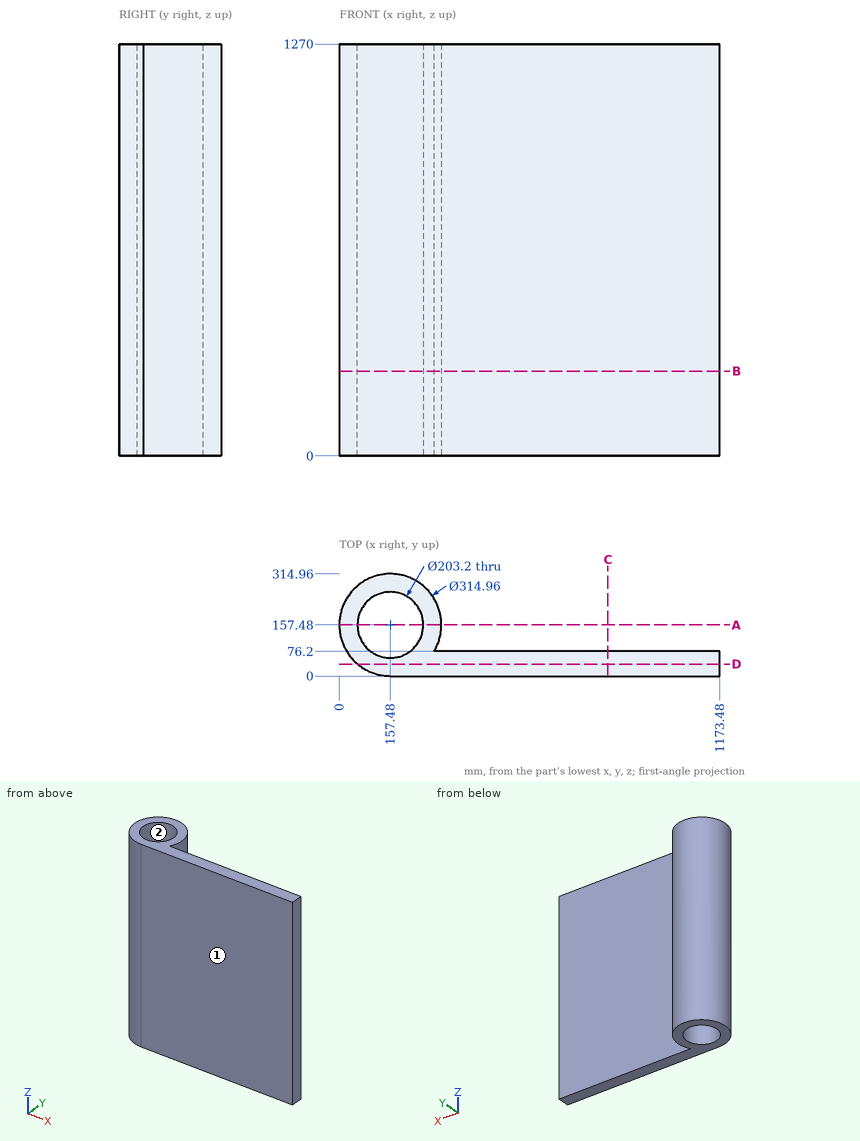
Here's the drawing with two shaded views (mm, measured from the low corner). I have some questions. Coordinates: 2 decimals unless noted, no trailing zeros. Order: outer loops, then holes, each group sorted by start corner. A loop starts at its lowest first (then second) coordinate and runs counter-clockwise, first axis right, second up.
Item 1: I need wall thicknesses on line 1 (X direction, y = 157, z = 430); line 2 (Y direction, x = 913, z = 977). Which ranges of each line are inside material? Lowest first, please.
Result sheet:
line 1: x = 0 to 55.88, 259.08 to 314.96
line 2: y = 0 to 76.2
Item 2: If we mould it in two halves opening along Y, with no side actions, what happens to the marked faces 1 and 2? For each: +Y half, -Y half, draft (parallel to the pull), parting line (faces both ways), or undercut.
Result sheet:
face 1: -Y half
face 2: undercut
Item 3: If we section it at A-A on y = 157.48: List the corners of the cut face in (x, z) for me.
Result sheet:
outline: (0, 0) - (55.88, 0) - (55.88, 1270) - (0, 1270) - close; (259.08, 0) - (314.96, 0) - (314.96, 1270) - (259.08, 1270) - close
Item 4: If we section it at B-B on z = 261: List the corners of the cut face in (x, y) for me, plus the area to 3 significant figures.
Result sheet:
outline: (157.48, 0) - (1173.48, 0) - (1173.48, 76.2) - (292.36, 76.2) arc R157.48 ccw (long way) to start; hole circle Ø203.2 at (157.48, 157.48)
area: 116,000 mm2
Item 5: If we section it at C-C on x = 828: List the corners of the cut face in (y, z) for me.
Result sheet:
outline: (0, 0) - (76.2, 0) - (76.2, 1270) - (0, 1270) - close
Item 6: For P1, Ø4, axis at y = 276.5, z = 695.5, coming from the +X side; P2, Ø12, axis at x = 799.5, z = 824, coming from the +Y side; P3, Ø6, axis at x = 250, y = 245.5, coming from the -Z side; P4, Ø3, axis at y = 252, z = 229, coming from the +X side, each with a flat end and sliding along its axis, tell me the tip position at first contact or that it passes through.
Result sheet:
P1: stops at x = 262.87
P2: stops at y = 76.2
P3: stops at z = 0
P4: stops at x = 284.55
Item 7: If we section it at D-D on y = 37: List the corners of the cut face in (x, z) for me.
Result sheet:
outline: (56.07, 0) - (1173.48, 0) - (1173.48, 1270) - (56.07, 1270) - close
